CAD build for the part. Positions are in the model's coordinates, mm. A direction names the side the tool comes from. Give positions to 0.01 mm unless a question says otherwise; leave off trailing zeros. Order: outer loops, then holes, each group sorted by start corner. A loop starts at its lowest first (then second) coordinate and runs counter-clockwise, first axis right, second up.
Item 1: Two-plate mould, pull along Z, no slides. Class faces 4 (the flat face through (-2, 430, -80)), 5 (the flat face through (555, -2, 63)), 6 (the flat face through (565, 2, 190)), 7 (the flat face through (2, 100, -30)): released by +Z, released by -Z, zero draft, split by the parting line, or undercut.
Item 2: Band-saw the part on A-A on y = -41.5. Give the cut face in (x, z).
Item 3: Wall check: L1, parallel to Y at x = 115.5, z = -38.5; L2, parallel to Y at x = 525, z = -74.75; L3, parallel to Y at x = 485, z = -65. Give the ranges that are in metal, low to high.
Item 4: Flat gauge pins, fed straight in: P1, Ø6, axis at x = 161, y = -49, coming from the +Z side; P2, Ø6, axis at y = 53.5, z = 122, coming from the -X side; P3, Ø4, axis at x = 43.5, y = -24, coming from the +Z side. Where does each tip first touch, or does it go through?
Item 5: Band-saw the part on B-B on z = -36.5. Give the cut face in (x, y), plus the area to 3 significant figures.
Item 6: Band-saw the part on C-C on x = -4.5. Give the cut face in (y, z), plus the area to 3 significant figures.
Item 7: Band-saw the part on D-D on y = -224.5. Give the cut face in (x, z), plus the area to 3 significant figures.
Item 8: Which spindle directions (+Z, -Z, +X, -X, +Y, -Y) get a long thin tool onto all of the face, cutting with end or side? Do faces 1 (the flat face through (-155, -6, 30)), 2 (the flat face through (-165, 6, 40)), 3 (the flat face through (-2, -410, -39)). Say none if no direction does.
```python
from build123d import *

# Parameters (mm, degrees)
F0_W      = 350
F0_H      = 900
F1_DEPTH  = 20
F2_W      = 100
F2_H      = 20
F3_DEPTH  = 175
F4_W      = 350
F4_H      = 40
F5_DEPTH  = 80
F6_W      = 20
F6_H      = 900
F7_DEPTH  = 20
F8_W      = 240
F8_H      = 20
F9_DEPTH  = 400
F10_W     = 20
F10_H     = 240
F11_DEPTH = 250
F12_R     = 5
F13_DEPTH = 20.001


# Not quite as in the source:
# - a pattern or mirror of a feature is missing from the dataset's text; its kind, count and spacing are read off the source's solid


with BuildPart() as f1:
    # F0 (on Top) → F1 (new body)
    with BuildSketch(Plane.XY):
        Rectangle(F0_W, F0_H)
    extrude(amount=F1_DEPTH)

    # F2 (on Right) → F3 (join, symmetric)
    with BuildSketch(Plane.YZ):
        Polygon((-100, 0), (-120, 0), (-120, -80), (-100, -80), (-100, -60), align=None)
        with Locations((-50, -70)):
            Rectangle(F2_W, F2_H)
    f3 = extrude(amount=F3_DEPTH, both=True)

    # F3_copies: F3 across plane
    add(f3.mirror(Plane.ZX))

    # F4 (on face) → F5 (join)
    with BuildSketch(Plane(origin=(0, 0, 0), x_dir=(1, 0, 0), z_dir=(0, 0, -1))):
        with Locations((0, 430)):
            Rectangle(F4_W, F4_H)
    f5 = extrude(amount=F5_DEPTH)

    # F5_copies: F5 across plane
    add(f5.mirror(Plane.ZX))

    # F6 (on face) → F7 (join)
    with BuildSketch(Plane.XY.offset(20)):
        with Locations((-165, 0)):
            Rectangle(F6_W, F6_H)
        with Locations((165, 0)):
            Rectangle(F6_W, F6_H)
    extrude(amount=F7_DEPTH)

    # F8 (on face) → F9 (join)
    with BuildSketch(Plane.YZ.offset(175)):
        with Locations((0, -70)):
            Rectangle(F8_W, F8_H)
    extrude(amount=F9_DEPTH)

    # F10 (on face) → F11 (join)
    with BuildSketch(Plane.XY.offset(-60)):
        with Locations((565, 0)):
            Rectangle(F10_W, F10_H)
    extrude(amount=F11_DEPTH)

    # F12 (on face) → F13 (cut, through all)
    with BuildSketch(Plane.XY.offset(-60)):
        with Locations((525, 90)):
            Circle(F12_R)
        with Locations((485, 0)):
            Circle(F12_R)
    extrude(amount=-F13_DEPTH, mode=Mode.SUBTRACT)


solid = f1.part
```
The answers:
1. face 4: released by -Z
1. face 5: zero draft
1. face 6: released by +Z
1. face 7: undercut
2. outline: (-175, -80) - (575, -80) - (575, 190) - (555, 190) - (555, -60) - (-175, -60) - close; (-175, 0) - (175, 0) - (175, 40) - (155, 40) - (155, 20) - (-155, 20) - (-155, 40) - (-175, 40) - close
3. L1: y = -450 to -410, -120 to -100, 100 to 120, 410 to 450
3. L2: y = -120 to 85, 95 to 120
3. L3: y = -120 to -5, 5 to 120
4. P1: stops at z = 40
4. P2: stops at x = 555
4. P3: stops at z = 20
5. outline: (-175, -450) - (175, -450) - (175, -410) - (-175, -410) - close; (-175, -120) - (175, -120) - (175, -100) - (-175, -100) - close; (-175, 100) - (175, 100) - (175, 120) - (-175, 120) - close; (-175, 410) - (175, 410) - (175, 450) - (-175, 450) - close; (555, -120) - (575, -120) - (575, 120) - (555, 120) - close
5. area: 46,800 mm2
6. outline: (-450, -80) - (-410, -80) - (-410, 0) - (-120, 0) - (-120, -80) - (120, -80) - (120, 0) - (410, 0) - (410, -80) - (450, -80) - (450, 20) - (-450, 20) - close; hole (-100, -60) - (100, -60) - (100, 0) - (-100, 0) - close
6. area: 31,600 mm2
7. outline: (-175, 0) - (175, 0) - (175, 40) - (155, 40) - (155, 20) - (-155, 20) - (-155, 40) - (-175, 40) - close
7. area: 7,800 mm2
8. face 1: +Z, +Y, -Y
8. face 2: +Z, -X, +Y, -Y
8. face 3: -Z, +X, -X
